Model file for the job. Use its own axes, mm. Give positions to 0.01 mm unless a question says otherwise; leave off trailing zeros. Order: outer loops, then holes, each group sorted by start corner. A loop starts at its lowest first (then second) coordinate and runs counter-clockwise, first axis right, second up. Notation, with made-up numbers: (34.5, -26) -> (88.5, -26) arc R18 ccw to (88.5, -4) -> close; hole circle Ø4 at (-3.5, 27.25). An arc over 180 degrees is marked (long way). Answer in a Markdown table with one row per item. Add a question column.
from build123d import *

# Parameters (mm, degrees)
F0_W     = 21.5
F0_H     = 21.5
F0_W_2   = 16
F0_H_2   = 16
F1_DEPTH = 237
F2_W     = 5
F2_H     = 30
F2_H_2   = 15
F3_DEPTH = 2.75
F4_W     = 16
F4_H     = 16
F5_DEPTH = 236
F6_W     = 16
F6_H     = 16
F7_DEPTH = 1


with BuildPart() as f1:
    # F0 (on Top) → F1 (new body)
    with BuildSketch(Plane.XY):
        with Locations((-10.75, 10.75)):
            Rectangle(F0_W, F0_H)
        with Locations((-10.75, 10.75)):
            Rectangle(F0_W_2, F0_H_2, mode=Mode.SUBTRACT)
        with Locations((-10.75, 10.75)):
            Rectangle(F0_W_2, F0_H_2)
    extrude(amount=F1_DEPTH)

    # F2 (on face) → F3 (cut)
    with BuildSketch(Plane.XZ):
        with Locations((-10.75, 221)):
            Rectangle(F2_W, F2_H)
        with Locations((-10.75, 146.5)):
            Rectangle(F2_W, F2_H_2)
        with Locations((-10.75, 131.5)):
            Rectangle(F2_W, F2_H_2)
        with Locations((-10.75, 57)):
            Rectangle(F2_W, F2_H)
    extrude(amount=-F3_DEPTH, mode=Mode.SUBTRACT)

    # F4 (on face) → F5 (cut)
    with BuildSketch(Plane(origin=(0, 0, 0), x_dir=(1, 0, 0), z_dir=(0, 0, -1))):
        with Locations((-10.75, -10.75)):
            Rectangle(F4_W, F4_H)
    extrude(amount=-F5_DEPTH, mode=Mode.SUBTRACT)

    # F6 (on face) → F7 (join)
    with BuildSketch(Plane(origin=(0, 0, 0), x_dir=(1, 0, 0), z_dir=(0, 0, -1))):
        with Locations((-10.75, -10.75)):
            Rectangle(F6_W, F6_H)
    extrude(amount=-F7_DEPTH)


solid = f1.part
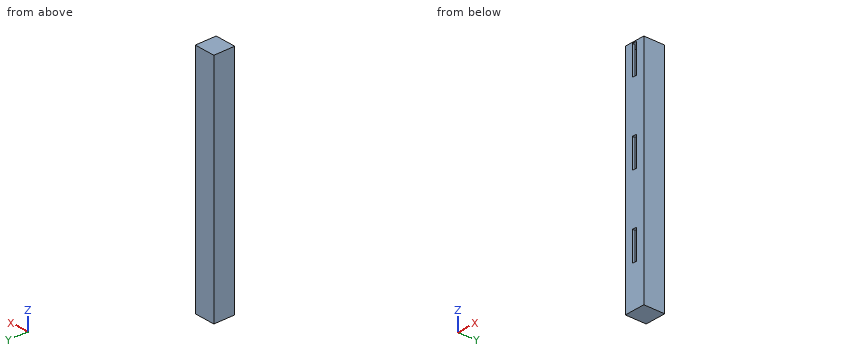
Item 1: Wall check: line 1 (Z direction, x = -9.25, y = 2); line 2 (X direction, y = 10.5, z = 196.5); line 3 (Z direction, x = -6.5, y = 16). Give the ranges that are in metal, low to high.
Item 2: Saw through at A-A on z = 83. List the corners of the cut face in (x, y), plus the area to 3 significant figures.
Item 3: Saw through at C-C on y = 7. List the corners of the cut face in (x, z), plus the area to 3 significant figures.
Item 4: Saw through at B-B on x = -10.25. List the corners of the cut face in (y, z).
Item 5: Saw through at D-D on z = 208.5. List the corners of the cut face in (x, y).
Evaluation:
| question | item | result |
|---|---|---|
| 1 | line 1 | z = 0 to 42, 72 to 124, 154 to 206, 236 to 237 |
| 1 | line 2 | x = -21.5 to -18.75, -2.75 to 0 |
| 1 | line 3 | z = 0 to 1, 236 to 237 |
| 2 | outline | (-21.5, 0) -> (0, 0) -> (0, 21.5) -> (-21.5, 21.5) -> close; hole (-18.75, 2.75) -> (-2.75, 2.75) -> (-2.75, 18.75) -> (-18.75, 18.75) -> close |
| 2 | area | 206 mm2 |
| 3 | outline | (-21.5, 0) -> (0, 0) -> (0, 237) -> (-21.5, 237) -> close; hole (-18.75, 1) -> (-2.75, 1) -> (-2.75, 236) -> (-18.75, 236) -> close |
| 3 | area | 1,340 mm2 |
| 4 | outline | (0, 0) -> (21.5, 0) -> (21.5, 237) -> (0, 237) -> (0, 236) -> (18.75, 236) -> (18.75, 1) -> (2.75, 1) -> (2.75, 42) -> (0, 42) -> close; (0, 72) -> (2.75, 72) -> (2.75, 124) -> (0, 124) -> close; (0, 154) -> (2.75, 154) -> (2.75, 206) -> (0, 206) -> close |
| 5 | outline | (-21.5, 0) -> (-13.25, 0) -> (-13.25, 2.75) -> (-18.75, 2.75) -> (-18.75, 18.75) -> (-2.75, 18.75) -> (-2.75, 2.75) -> (-8.25, 2.75) -> (-8.25, 0) -> (0, 0) -> (0, 21.5) -> (-21.5, 21.5) -> close |
